Geometry check sheet. Reference: the model listing, model coordinates, mm. Face numbers are marked on the shaded views. A direction names the side the tool comes from. Give positions to 0.01 mm unless a question says otherwise; leave off trailing zeros. Loops run counter-clockwise (first coordinate to the right, second up) from the corner with the lowest first, then second, coordinate; pieces in that order, holes last. Notation, with made-up numbers: (-5.5, 34) -> (31.5, 34) arc R18 ccw to (31.5, 54) -> close; hole circle Ø1 at (64, -26.75). An arc over 180 degrees is marked (long way). Answer as a JSON object with one key per item and string values.
from build123d import *

# Parameters (mm, degrees)
F1_DEPTH = 3
F3_DEPTH = 3


with BuildPart() as f1:
    # F0 (on Top) → F1 (new body)
    with BuildSketch(Plane.XY):
        with BuildLine():
            ThreePointArc((10, 10), (0, 0), (10, -10))
            Line((10, -10), (10, -2.3114))
            ThreePointArc((10, -2.3114), (7.6886, 0), (10, 2.3114))
            Line((10, 2.3114), (10, 10))
        make_face()
        with BuildLine():
            Line((-10, -10), (10, -10))
            ThreePointArc((10, -10), (0, 0), (10, 10))
            Line((10, 10), (-10, 10))
            Line((-10, 10), (-10, -10))
        make_face()
        with BuildLine():
            Line((10, -2.3114), (10, -10))
            ThreePointArc((10, -10), (17.0710678119, -7.0710678119), (20, 0))
            ThreePointArc((20, 0), (17.0710678119, 7.0710678119), (10, 10))
            Line((10, 10), (10, 2.3114))
            ThreePointArc((10, 2.3114), (11.634406614, 1.634406614), (12.3114, 0))
            ThreePointArc((12.3114, 0), (11.634406614, -1.634406614), (10, -2.3114))
        make_face()
    extrude(amount=F1_DEPTH)

    # F2 (on face) → F3 (join)
    with BuildSketch(Plane(origin=(-10, 0, 0), x_dir=(0, -1, 0), z_dir=(-1, 0, 0))):
        with BuildLine():
            Line((-10, 20), (-10, 0))
            Line((-10, 0), (10, 0))
            Line((10, 0), (10, 20))
            ThreePointArc((10, 20), (0, 10), (-10, 20))
        make_face()
        with BuildLine():
            ThreePointArc((10, 20), (0, 30), (-10, 20))
            Line((-10, 20), (-2.3114, 20))
            ThreePointArc((-2.3114, 20), (0, 22.3114), (2.3114, 20))
            Line((2.3114, 20), (10, 20))
        make_face()
        with BuildLine():
            Line((-2.3114, 20), (-10, 20))
            ThreePointArc((-10, 20), (0, 10), (10, 20))
            Line((10, 20), (2.3114, 20))
            ThreePointArc((2.3114, 20), (0, 17.6886), (-2.3114, 20))
        make_face()
    extrude(amount=-F3_DEPTH)


solid = f1.part
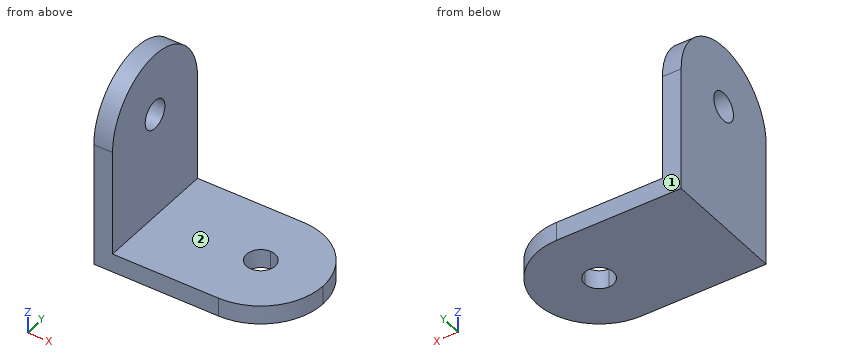
1) Section check A-A on x = 9.5. Record the cut outline in (y, z), plus the area to 3 significant figures.
Geometry check:
{"outline": "(-10, 0) -> (-2.26, 0) -> (-2.26, 3) -> (-10, 3) -> close; (2.26, 0) -> (10, 0) -> (10, 3) -> (2.26, 3) -> close", "area": "46.5 mm2"}
2) Section check C-C on z = 18.5. Record the cut outline in (x, y).
Geometry check:
{"outline": "(-10, -10) -> (-7, -10) -> (-7, -1.76) -> (-10, -1.76) -> close; (-10, 1.76) -> (-7, 1.76) -> (-7, 10) -> (-10, 10) -> close"}
3) Material ranges on line 1 along Z through (x, y) = (-9.15, 0); line 2 along Z through (x, y) = (-5.5, 8.5); line 3 along X through (y, z) = (3.25, 17.5), recorded low to high. Write a range as from..to.
Geometry check:
{"line 1": "z = 0..17.69, 22.31..30", "line 2": "z = 0..3", "line 3": "x = -10..-7"}
4) Section check D-D on y = -1.5. Record the cut outline in (x, z).
Geometry check:
{"outline": "(-10, 0) -> (8.24, 0) -> (8.24, 3) -> (-7, 3) -> (-7, 18.24) -> (-10, 18.24) -> close; (-10, 21.76) -> (-7, 21.76) -> (-7, 29.89) -> (-10, 29.89) -> close; (11.76, 0) -> (19.89, 0) -> (19.89, 3) -> (11.76, 3) -> close"}
5) Depth check by flat-ended pin: P1, Ø4, axis at x = -1, y = -5, coming from the +Z side; P2, Ø7.5, axis at y = 0, z = 20, coming from the +X side. Enter the tip coordinate at first touch or a pass-through.
Geometry check:
{"P1": "stops at z = 3", "P2": "stops at x = -7"}
6) Section check B-B on y = 6. Record the cut outline in (x, z), plus the area to 3 significant figures.
Geometry check:
{"outline": "(-10, 0) -> (18, 0) -> (18, 3) -> (-7, 3) -> (-7, 28) -> (-10, 28) -> close", "area": "159 mm2"}
7) Tool access check on the marked faces 1 and 2. Record the directions out of +Z, -Z, +X, -X, +Y, -Y that give a thin tool (end or side, any length) a straight path to the whole face; none if there is none.
Geometry check:
{"face 1": "+Z, -Z, +X, -X, +Y", "face 2": "+Z, +X, +Y, -Y"}
